Geometry: final body of the model. Coordinates: model frame, mm. Face numbers are marked on the shaded views. A direction names the side the tool comes from. Give positions to 0.01 mm unless a question says otherwise; leave off trailing zeros. Write each loop counter-clockwise with the first axis right and the second up, starting at its lowest first coordinate (ties: lowest second). Pieces come first, ordered by that corner, then holes. Notation, with made-up numbers: (27.25, -2.5) -> (54.25, -2.5) arc R29 cw to (54.25, 28.5) -> close; hole circle Ø1 at (70, 4.25). An arc over 180 degrees is marked (long way). Answer as a JSON object with one key per item and string values.
from build123d import *

# Parameters (mm, degrees)
SKETCH_W              = 25
SKETCH_H              = 25
PAD_DEPTH             = 5
SKETCH001_R           = 7.5
PAD001_DEPTH          = 40
SKETCH004_R           = 4
POCKET_DEPTH          = 45.001
SKETCH005_R           = 3
POCKET001_DEPTH       = 3.1
POLARPATTERN_COUNT    = 4
SKETCH006_R           = 1.75
POCKET002_DEPTH       = 156.356231
POLARPATTERN001_COUNT = 4
CHAMFER_SIZE          = 1.5
CHAMFER001_SIZE       = 0.2
FILLET_R              = 0.2


with BuildPart() as part:
    # Sketch → Pad (new body)
    with BuildSketch(Plane.XY):
        Rectangle(SKETCH_W, SKETCH_H)
    extrude(amount=PAD_DEPTH)

    # Sketch001 (on Face6 of Pad) → Pad001 (join)
    with BuildSketch(Plane.XY.offset(5)):
        Circle(SKETCH001_R)
    extrude(amount=PAD001_DEPTH)

    # Sketch004 (on Face4 of Pad001) → Pocket (cut, through all)
    with BuildSketch(Plane(origin=(0, 0, 0), x_dir=(1, 0, 0), z_dir=(0, 0, -1))):
        Circle(SKETCH004_R)
    extrude(amount=-POCKET_DEPTH, mode=Mode.SUBTRACT)

    # Sketch005 (on Face4 of Pocket) → Pocket001 (cut)
    with BuildSketch(Plane(origin=(0, 0, 0), x_dir=(1, 0, 0), z_dir=(0, 0, -1))):
        with Locations((-8.485281, 8.485281)):
            Circle(SKETCH005_R)
    pocket001 = extrude(amount=-POCKET001_DEPTH, mode=Mode.SUBTRACT)

    # PolarPattern: Pocket001 ×4 about axis
    polarpattern_axis = Axis((0, 0, 0), (0, 0, -1))
    for i in range(1, POLARPATTERN_COUNT):
        add(pocket001.rotate(polarpattern_axis, i * 360 / POLARPATTERN_COUNT), mode=Mode.SUBTRACT)

    # Sketch006 (on Face16 of PolarPattern) → Pocket002 (cut, through all)
    with BuildSketch(Plane(origin=(0, 0, 3.1), x_dir=(1, 0, 0), z_dir=(0, 0, -1))):
        with Locations((-8.485281, 8.485281)):
            Circle(SKETCH006_R)
    pocket002 = extrude(amount=-POCKET002_DEPTH, mode=Mode.SUBTRACT)

    # PolarPattern001: Pocket002 ×4 about axis
    polarpattern001_axis = Axis((0, 0, 3.1), (0, 0, -1))
    for i in range(1, POLARPATTERN001_COUNT):
        add(pocket002.rotate(polarpattern001_axis, i * 360 / POLARPATTERN001_COUNT), mode=Mode.SUBTRACT)

    # Chamfer
    chamfer_edges = [part.edges().sort_by_distance(p)[0] for p in [
        (-12.5, 12.5, 2.5),
        (-12.5, -12.5, 2.5),
        (12.5, -12.5, 2.5),
        (12.5, 12.5, 2.5),
    ]]
    chamfer(chamfer_edges, length=CHAMFER_SIZE)

    # Chamfer001
    chamfer001_edges = [part.edges().sort_by_distance(p)[0] for p in [
        (-11.75, 11.75, 0),
        (0, 12.5, 0),
        (11.75, 11.75, 0),
        (12.5, 0, 0),
        (11.75, -11.75, 0),
        (0, -12.5, 0),
        (-11.75, -11.75, 0),
        (-12.5, 0, 0),
        (-11.75, 11.75, 5),
        (0, 12.5, 5),
        (11.75, 11.75, 5),
        (12.5, 0, 5),
        (0, -12.5, 5),
        (-11.75, -11.75, 5),
        (-12.5, 0, 5),
        (11.75, -11.75, 5),
    ]]
    chamfer(chamfer001_edges, length=CHAMFER001_SIZE)

    # Fillet
    fillet_edges = [part.edges().sort_by_distance(p)[0] for p in [
        (-7.5, 0, 45),
    ]]
    fillet(fillet_edges, radius=FILLET_R)


solid = part.part
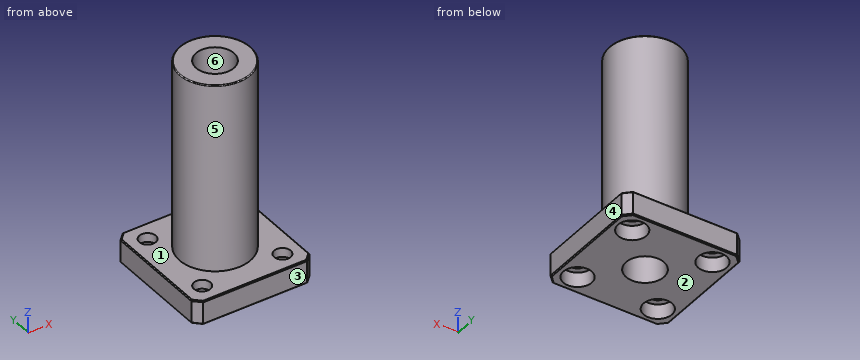
Q1. Cut plane A-A (y = 0). Return the cut outline in (x, z), and give its area (3 significant figures).
Values:
{"outline": "(-12.5, 0.2) -> (-12.3, 0) -> (-4, 0) -> (-4, 45) -> (-7.3, 45) arc R0.2 ccw to (-7.5, 44.8) -> (-7.5, 5) -> (-12.3, 5) -> (-12.5, 4.8) -> close; (4, 0) -> (12.3, 0) -> (12.5, 0.2) -> (12.5, 4.8) -> (12.3, 5) -> (7.5, 5) -> (7.5, 44.8) arc R0.2 ccw to (7.3, 45) -> (4, 45) -> close", "area": "365 mm²"}
Q2. Cut plane D-D (z = 33). Return the cut outline in (x, y), and give its area (3 significant figures).
Values:
{"outline": "circle Ø15 at (0, 0); hole circle Ø8 at (0, 0)", "area": "126 mm²"}
Q3. Mould query, pull axis Y, two halves, no side actions, for the marked faces 3, 4, 5 and 6. Classes: pulls with the +Y half, pulls with the -Y half, needs draft (parallel to the pull), parting line crosses it, or undercut.
Values:
{"face 3": "pulls with the -Y half", "face 4": "needs draft", "face 5": "parting line crosses it", "face 6": "undercut"}
Q4. Set-up query: the marked faces 1 and 2. Return all of +Z, -Z, +X, -X, +Y, -Y with unobstructed straight access to the full face (end or side cutting, diameter ignored); none if empty.
Values:
{"face 1": "+Z", "face 2": "-Z, +X, -X, +Y, -Y"}
Q5. Material intervals for L1, parallel to Z at x = 7.5, y = -6; L2, parallel to Y at x = 10, z = 4; L3, parallel to Z at x = -4.25, y = 7.5, sorted ascending. Write a range as from..to.
Values:
{"L1": "3.1..5", "L2": "-12.5..-9.36, -7.61..7.61, 9.36..12.5", "L3": "0..5"}
Q6. First-contact query: P1, Ø5.5, axis at x = -8.49, y = -8.49, coming from the +Z side; P2, Ø7, axis at x = 0, y = 0, coming from the -Z side; P3, Ø3, axis at x = -9.5, y = -8.5, coming from the -Z side; P4, Ø4, axis at x = -2.5, z = 11, coming from the -Y side. Flat tips, straight axial feed; report the tip coordinate or a pass-through.
Values:
{"P1": "z = 5", "P2": "through", "P3": "z = 3.1", "P4": "y = -7.48"}
Q7. Cut plane C-C (y = -8). Return the cut outline in (x, z).
Values:
{"outline": "(-12.5, 0.2) -> (-12.3, 0) -> (-11.45, 0) -> (-11.45, 3.1) -> (-10.17, 3.1) -> (-10.17, 5) -> (-12.3, 5) -> (-12.5, 4.8) -> close; (-6.8, 3.1) -> (-5.52, 3.1) -> (-5.52, 0) -> (5.52, 0) -> (5.52, 3.1) -> (6.8, 3.1) -> (6.8, 5) -> (-6.8, 5) -> close; (10.17, 3.1) -> (11.45, 3.1) -> (11.45, 0) -> (12.3, 0) -> (12.5, 0.2) -> (12.5, 4.8) -> (12.3, 5) -> (10.17, 5) -> close"}
